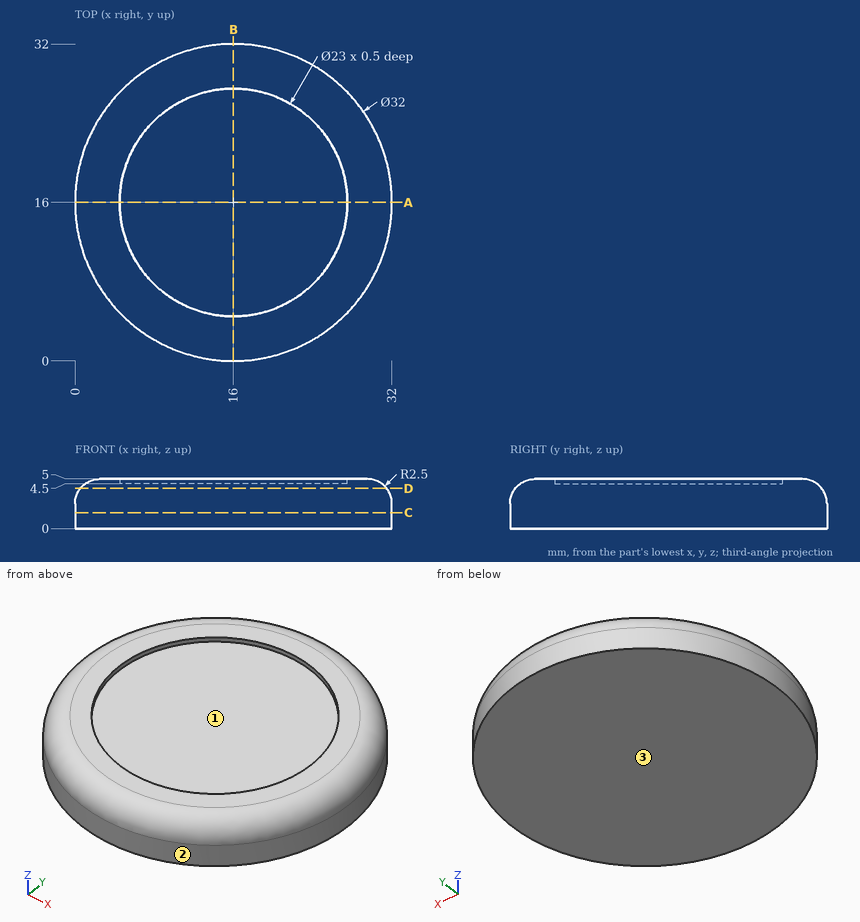
Geometry: see drawing. Coordinates: mm, zero at the bounding-box minimum. Give positions to 0.01 mm unless a question says otherwise; leave off trailing zeros. Loops run counter-clockwise (first coordinate to the right, second up) from the corner with the lowest first, then second, coordinate; pieces in that order, holes last. Notation, with made-up numbers: (61.25, 29) -> (120.25, 29) arc R30 cw to (120.25, 56) -> close; hole circle Ø5 at (-35, 13.5). An arc over 180 degrees is marked (long way). Answer as a JSON object with one key per item and string values. Group by question number.
Item 1: Pull-direction query (Y, two-part tool) for the marked faces 1, 2 and 3; classes: released by +Y, released by -Y, zero draft, split by the parting line, or undercut.
Item 2: Line query: probe 1 along Z at (x, y) = (16.5, 11); probe 2 along Y at (x, z) = (16, 4.8); probe 3 along Y at (x, z) = (14.5, 1.85). Output: solid intervals per line, ascending.
Item 3: Pin query (flat end, axial travel): P1, Ø1.5, axis at x = 13.5, y = 27, coming from the +Z side; P2, Ø1, axis at x = 9, z = 4, coming from the -Y side; P3, Ø1, axis at x = 13, z = 2, coming from the +Y side; P4, Ø11.5, axis at x = 12.5, y = 15, coming from the +Z side. Return the tip coordinate at first contact, or that it passes through.
Item 4: Cut plane A-A, the plane y = 16. Return the cut outline in (x, z), and give its area (3 significant figures).
Item 5: Cut plane C-C, the plane z = 1.6. Return the cut outline in (x, y), and give its area (3 significant figures).
Item 6: Cut plane D-D, the plane z = 4.05. Return the cut outline in (x, y).
Checks:
{
 "1": {"face 1": "undercut", "face 2": "split by the parting line", "face 3": "zero draft"},
 "2": {"probe 1": "z = 0 to 4.5", "probe 2": "y = 1.52 to 4.5, 27.5 to 30.48", "probe 3": "y = 0.07 to 31.93"},
 "3": {"P1": "stops at z = 5", "P2": "stops at y = 1.75", "P3": "stops at y = 31.8", "P4": "stops at z = 4.5"},
 "4": {"outline": "(0, 0) -> (32, 0) -> (32, 2.5) arc R2.5 ccw to (29.5, 5) -> (27.5, 5) -> (27.5, 4.5) -> (4.5, 4.5) -> (4.5, 5) -> (2.5, 5) arc R2.5 ccw to (0, 2.5) -> close", "area": "146 mm²"},
 "5": {"outline": "circle Ø32 at (16, 16)", "area": "804 mm²"},
 "6": {"outline": "circle Ø30.92 at (16, 16)"}
}
